CAD build for the part. Positions are in the model's coordinates, mm. Give positions to 0.01 mm unless a question says otherwise; leave off trailing zeros. Loops run counter-clockwise (first coordinate to the right, second up) from the corner with the lowest first, then second, coordinate; pieces in that order, holes last. Notation, with made-up numbers: (67.5, 11) - (88.5, 11) arc R34 ccw to (88.5, 48) - close; hole circle Ø7 at (15.5, -39.5). An arc over 180 degrees is marked (long way). Return JSON: item names as keys, results as strings.
from build123d import *

# Parameters (mm, degrees)
EXTRUDE_1_DEPTH     = 3
SKETCH_5_R          = 2
SKETCH_5_R_2        = 2.5
SKETCH_5_W          = 40
SKETCH_5_H          = 60
CUT_EXTRUDE_1_DEPTH = 3


with BuildPart() as part:
    # 草图4 → 凸台-拉伸1 (new body)
    with BuildSketch(Plane(origin=(0, 0, 0), x_dir=(1, 0, 0), z_dir=(0, 1, 0))):
        Polygon((10, 0), (0, 0), (0, -19), (-3, -19), (-3, -49), (0, -49), (0, -69), (-3, -69), (-3, -99), (0, -99), (0, -118), (10, -118), (10, -121), (40, -121), (40, -118), (60, -118), (60, -121), (90, -121), (90, -118), (110, -118), (110, -121), (140, -121), (140, -118), (160, -118), (160, -121), (190, -121), (190, -118), (210, -118), (210, -121), (240, -121), (240, -118), (260, -118), (260, -121), (290, -121), (290, -118), (300, -118), (300, 0), (290, 0), (290, 3), (260, 3), (260, 0), (240, 0), (240, 3), (210, 3), (210, 0), (190, 0), (190, 3), (160, 3), (160, 0), (140, 0), (140, 3), (110, 3), (110, 0), (90, 0), (90, 3), (60, 3), (60, 0), (40, 0), (40, 3), (10, 3), align=None)
    extrude(amount=-EXTRUDE_1_DEPTH)

    # 草图5 → 切除-拉伸1 (cut)
    with BuildSketch(Plane(origin=(0, 0, 0), x_dir=(1, 0, 0), z_dir=(0, 1, 0))):
        with Locations((295, -96)):
            Circle(SKETCH_5_R)
        with Locations((295, -81)):
            Circle(SKETCH_5_R)
        with Locations((295, -22)):
            Circle(SKETCH_5_R)
        with Locations((295, -37)):
            Circle(SKETCH_5_R)
        with Locations((35, -24)):
            Circle(SKETCH_5_R_2)
        with Locations((35, -94)):
            Circle(SKETCH_5_R_2)
        with Locations((85, -94)):
            Circle(SKETCH_5_R_2)
        with Locations((85, -24)):
            Circle(SKETCH_5_R_2)
        with Locations((60, -59)):
            Rectangle(SKETCH_5_W, SKETCH_5_H)
    extrude(amount=-CUT_EXTRUDE_1_DEPTH, mode=Mode.SUBTRACT)


solid = part.part
1. Drill centre lines: probe 1 along Z at (x, y) = (85, -2.15); probe 2 along Z at (x, y) = (295, -1.7); probe 3 along X at (y, z) = (-1.55, 64.5). Where is each one in solid material? Low to high.
Values follow:
{"probe 1": "z = -3 to 21.5, 26.5 to 91.5, 96.5 to 121", "probe 2": "z = 0 to 20, 24 to 35, 39 to 79, 83 to 94, 98 to 118", "probe 3": "x = 0 to 40, 80 to 300"}
2. Cut at A-A, the plane x = 43. Write the cut outline in (y, z).
Values follow:
{"outline": "(-3, 0) - (0, 0) - (0, 29) - (-3, 29) - close; (-3, 89) - (0, 89) - (0, 118) - (-3, 118) - close"}
3. Drop flat-ended pins along their axis: P1, Ø0.9, axis at x = -1.5, y = -1, coming from the +Z side; P2, Ø0.9, axis at x = 6.5, y = -1, coming from the -Z side; P3, Ø0.9, axis at x = 51.5, y = -1, coming from the +Z side; P4, Ø3, axis at x = 85, z = 24, coming from the -Y side. Give the stop position or say it passes through.
Values follow:
{"P1": "stops at z = 99", "P2": "stops at z = 0", "P3": "stops at z = 118", "P4": "passes through"}
4. Pull direction X, two halves, no side cores. Call faces 1 (the face through (146, -3, 58)), 2 (the face through (84.67, -1.48, 91.52)): +X half, -X half, draft (parallel to the pull), parting line (faces both ways), or undercut.
Values follow:
{"face 1": "draft", "face 2": "undercut"}
5. Cut at B-B, the plane y = -1.25. Give the number of separate pieces and of enclosed holes in the cut face, plus the area to 3 significant figures.
Values follow:
{"separate pieces": "1", "enclosed holes": "9", "area": "34,100 mm²"}
